Here's how the part is built. I have some questions about the finished solid (model axes, mm). A direction names the side the tool comes from. Round coordinates to 2 decimals unless told otherwise and drop trailing zeros. Write each loop counter-clockwise with the first axis right and the second up, starting at its lowest first coordinate (ties: lowest second). Pieces come first, ordered by that corner, then holes. Notation, with made-up numbers: (54.25, 55) -> (107.25, 55) arc R30 ccw to (107.25, 87) -> close; hole circle Ø9 at (-15.5, 11.5). An arc over 180 degrees is marked (long way). Answer as CSV lines item,"result".
```python
from build123d import *

# Parameters (mm, degrees)
CUT_EXTRUDE1_DEPTH      = 23.315913604
CUT_EXTRUDE1_DEPTH_BACK = 23.315913604
CUT_EXTRUDE2_START      = -8
CUT_EXTRUDE2_DEPTH      = 8
CUT_EXTRUDE3_REACH      = 26.886
SKETCH4_R               = 1.9
CUT_EXTRUDE4_START      = -5.7
SKETCH5_R               = 2.55
CUT_EXTRUDE4_DEPTH      = 5.7


with BuildPart() as part:
    # Sketch2 → Revolve1 (revolve)
    with BuildSketch(Plane(origin=(0, 0, 0), x_dir=(0, 0, -1), z_dir=(1, 0, 0))):
        Polygon((0, 0), (-20, 0), (-20, 6.5), (-12, 6.5), (-12, 7), (-11, 7), (-9, 5), (-1, 5), (-1, 7), (0, 7), align=None)
    revolve(axis=Axis((0, 0, 0), (0, 0, 1)))

    # Sketch1 → Cut-Extrude1 (cut, two sides: drawn at the far end of the back side and taken through both)
    with BuildSketch(Plane.XY.offset(-CUT_EXTRUDE1_DEPTH_BACK)):
        with BuildLine():
            Line((-2.05, 1.516575089), (-2.05, -1.516575089))
            ThreePointArc((-2.05, -1.516575089), (2.55, 0), (-2.05, 1.516575089))
        make_face()
    extrude(amount=CUT_EXTRUDE1_DEPTH + CUT_EXTRUDE1_DEPTH_BACK, mode=Mode.SUBTRACT)

    # Sketch3 → Cut-Extrude2 (cut)
    with BuildSketch(Plane.XY.offset(20).offset(CUT_EXTRUDE2_START)):
        with BuildLine():
            Line((-6.05, -2.376446928), (-6.05, 2.376446928))
            ThreePointArc((-6.05, 2.376446928), (-6.5, 0), (-6.05, -2.376446928))
        make_face()
    extrude(amount=CUT_EXTRUDE2_DEPTH, mode=Mode.SUBTRACT)

    # Sketch4 → Cut-Extrude3 (cut, up to next)
    with BuildSketch(Plane.ZY.offset(6.05), mode=Mode.PRIVATE) as cut_extrude3_sk1:
        with Locations((14.3, 0)):
            Circle(SKETCH4_R)
    cut_extrude3_tool1 = extrude(cut_extrude3_sk1.sketch, amount=-CUT_EXTRUDE3_REACH, mode=Mode.PRIVATE) & part.part
    add(cut_extrude3_tool1.solids().sort_by_distance((-6.05, 0, 14.3))[0], mode=Mode.SUBTRACT)

    # Sketch5 → Cut-Extrude4 (cut)
    with BuildSketch(Plane.XY.offset(20).offset(CUT_EXTRUDE4_START)):
        with Locations(Location((0, 0, 0), (0, 0, 143.5062334))):
            Circle(SKETCH5_R)
    extrude(amount=CUT_EXTRUDE4_DEPTH, mode=Mode.SUBTRACT)


solid = part.part
```
1. Suppose I cut it at C-C on z = 4. Please give me the cut outline in (x, y).
Numbers:
outline,"circle Ø10 at (0, 0); hole (-2.05, -1.52) arc R2.55 ccw (long way) to (-2.05, 1.52) -> close"
2. On a 3-axis mill with a long thin cutter (end or side, diameter ignored), from which of +Z, -Z, +X, -X, +Y, -Y can I reach the whole of each face in a straight line? I mean faces 4 (the face through (-3.906, -1.156, 12.792)), 5 (the face through (-6.3, 0, 12)), 6 (the face through (-5, 2, 1)), 7 (the face through (-6.05, 0, 17)). Say none if no direction works.
Numbers:
face 4,"-X"
face 5,"+Z"
face 6,"none"
face 7,"+Z, -X, +Y, -Y"
3. For pin 1 Ø3 at (y, z) = (5, 11) entering from +X; pin 2 Ø3.5 at (y, z) = (0, 6.5) entering from +X; pin 3 Ø3 at (y, z) = (0, 14.3) entering from +X, each with a flat end and sliding along its axis, tell me the tip position at first contact or that it passes through.
Numbers:
pin 1,"stops at x = 6.06"
pin 2,"stops at x = 5"
pin 3,"stops at x = 6.5"
4. If we mould it in two halves opening along X, with no side actions, what happens to faces 1 (the face through (-2.05, 0, 6)), 2 (the face through (6.495, -0.252, 15.944)), 3 (the face through (-3, 0, 20))? For each: released by +X, released by -X, zero draft, split by the parting line, or undercut.
Numbers:
face 1,"undercut"
face 2,"split by the parting line"
face 3,"zero draft"
5. Suppose I cut it at B-B on y = 0. Please give me the cut outline in (x, z).
Numbers:
outline,"(-7, 0) -> (-2.05, 0) -> (-2.05, 12.4) -> (-6.05, 12.4) -> (-6.05, 12) -> (-7, 12) -> (-7, 11) -> (-5, 9) -> (-5, 1) -> (-7, 1) -> close; (-6.05, 16.2) -> (-2.55, 16.2) -> (-2.55, 20) -> (-6.05, 20) -> close; (2.55, 0) -> (7, 0) -> (7, 1) -> (5, 1) -> (5, 9) -> (7, 11) -> (7, 12) -> (6.5, 12) -> (6.5, 20) -> (2.55, 20) -> close"
6. If I drill on line 1 (Y direction, x = 0, z = 12.5); line 2 (Z direction, x = 0.25, y = 6.75); line 3 (Y direction, x = -3.9, z = 14.3), over which ranges is the centre line in solid material (lowest first)?
Numbers:
line 1,"y = -6.5 to -2.55, 2.55 to 6.5"
line 2,"z = 0 to 1, 10.75 to 12"
line 3,"y = -5.2 to -1.9, 1.9 to 5.2"
7. Suppose I cut it at D-D on z = 14.3. Please give me the cut outline in (x, y), and give its area (3 significant figures).
Numbers:
outline,"(-6.05, -2.38) arc R6.5 ccw (long way) to (-6.05, 2.38) -> (-6.05, 1.9) -> (-1.7, 1.9) arc R2.55 cw (long way) to (-1.7, -1.9) -> (-6.05, -1.9) -> close"
area,"96.6 mm^2"
8. Suppose I cut it at A-A on x = 0. Please give me the cut outline in (y, z), and give its area (3 significant figures).
Numbers:
outline,"(-7, 0) -> (-2.55, 0) -> (-2.55, 20) -> (-6.5, 20) -> (-6.5, 12) -> (-7, 12) -> (-7, 11) -> (-5, 9) -> (-5, 1) -> (-7, 1) -> close; (2.55, 0) -> (7, 0) -> (7, 1) -> (5, 1) -> (5, 9) -> (7, 11) -> (7, 12) -> (6.5, 12) -> (6.5, 20) -> (2.55, 20) -> close"
area,"134 mm^2"
